Build history of the part. All positions in model axes, mm. A direction names the side the tool comes from. Round coordinates to 2 decimals unless told otherwise and drop trailing zeros. Write each loop counter-clockwise with the first axis right and the second up, starting at its lowest first coordinate (ties: lowest second). Pieces come first, ordered by that corner, then holes. Notation, with made-up numbers: M -5.5,14 L 0.5,14 A7 ccw 0.5,24 Z; hole C -4.5,-24 d3. An arc over 180 degrees is marked long. Write item = value, one per line.
from build123d import *

# Parameters (mm, degrees)
F0_W     = 55
F0_H     = 25
F0_R     = 4
F0_W_2   = 20
F0_H_2   = 20
F0_R_2   = 7.5
F1_DEPTH = 5


with BuildPart() as f1:
    # F0 (on Top) → F1 (new body)
    with BuildSketch(Plane.XY):
        with Locations((12.5, 0)):
            Rectangle(F0_W, F0_H)
        with Locations((32.434259, -6.458126)):
            Circle(F0_R, mode=Mode.SUBTRACT)
        Rectangle(F0_W_2, F0_H_2, mode=Mode.SUBTRACT)
        with Locations((20.582465, 2.502987)):
            Circle(F0_R_2, mode=Mode.SUBTRACT)
    extrude(amount=F1_DEPTH)


solid = f1.part
1. Flat gauge pin, fed straight in: pin 1 (4 mm diameter, centred on x = 4.5, y = -7.5, fed in from +Z). Where does the tip first touch, or does it go through?
Responses:
pin_1 = through
2. Band-saw the part on A-A (x = 2). List the corners of the cut face in (y, z).
Responses:
outline = M -12.5,0 L -10,0 L -10,5 L -12.5,5 Z; M 10,0 L 12.5,0 L 12.5,5 L 10,5 Z
3. Band-saw the part on B-B (y = 3). List the corners of the cut face in (x, z).
Responses:
outline = M -15,0 L -10,0 L -10,5 L -15,5 Z; M 10,0 L 13.1,0 L 13.1,5 L 10,5 Z; M 28.07,0 L 40,0 L 40,5 L 28.07,5 Z
4. Band-saw the part on C-C (z = 0.75). List the corners of the cut face in (x, y).
Responses:
outline = M -15,-12.5 L 40,-12.5 L 40,12.5 L -15,12.5 Z; hole M -10,-10 L 10,-10 L 10,10 L -10,10 Z; hole C 20.58,2.5 d15; hole C 32.43,-6.46 d8
5. Mould opens along X. For faces 3 (the face through (36.25, -5.26, 2.46)), 4 (the face through (12, 0, 5)), 5 (the face through (0, 10, 2)), 6 (the face through (-15, 0, 2)) say: pulls with the +X half, pulls with the -X half, needs draft (parallel to the pull), parting line crosses it, or undercut.
Responses:
face_3 = undercut
face_4 = needs draft
face_5 = undercut
face_6 = pulls with the -X half
6. Tool access for faces 1 (the face through (-10, 0, 2)), 2 (the face through (12, 12.5, 2)): list every direction of +Z, -Z, +X, -X, +Y, -Y with a clear straight run to the whole face (end or side of a thin tool).
Responses:
face_1 = +Z, -Z
face_2 = +Z, -Z, +X, -X, +Y
7. Probe probe 1 along Y at (x, z) = (6, 2.8); probe 2 along X at (y, z) = (-8.75, 3.85); probe 3 along X at (y, z) = (-7, 2). List the from-to ranges inside material, lowest first.
Responses:
probe_1 = -12.5 to -10, 10 to 12.5
probe_2 = -15 to -10, 10 to 29.16, 35.71 to 40
probe_3 = -15 to -10, 10 to 28.47, 36.4 to 40
8. Band-saw the part on D-D (x = 29.5). List the corners of the cut face in (y, z), plus the area to 3 significant figures.
Responses:
outline = M -12.5,0 L -9.18,0 L -9.18,5 L -12.5,5 Z; M -3.74,0 L 12.5,0 L 12.5,5 L -3.74,5 Z
area = 97.8 mm²
